from build123d import *

# Parameters (mm, degrees)
SKIZZE1_R                            = 33.5
AUFSATZ_LINEAR_AUSTRAGEN1_DEPTH      = 36
SKIZZE2_R                            = 19
AUFSATZ_LINEAR_AUSTRAGEN2_DEPTH      = 4.5
SKIZZE3_R                            = 13.25
AUFSATZ_LINEAR_AUSTRAGEN3_DEPTH      = 6
SKIZZE4_R                            = 13
AUFSATZ_LINEAR_AUSTRAGEN4_DEPTH      = 26
AUFSATZ_LINEAR_AUSTRAGEN4_DEPTH_BACK = 29
SKIZZE5_R                            = 20
AUFSATZ_LINEAR_AUSTRAGEN5_DEPTH      = 9
SKIZZE6_R                            = 31.75
AUFSATZ_LINEAR_AUSTRAGEN6_DEPTH      = 7
SKIZZE7_W                            = 58.3
SKIZZE7_H                            = 58.3
AUFSATZ_LINEAR_AUSTRAGEN7_DEPTH      = 7
F_10_0_10_DURCHMESSER_BOHRUNG1_D     = 10
F_10_0_10_DURCHMESSER_BOHRUNG1_DEPTH = 7
SKIZZE13_R                           = 19
AUFSATZ_LINEAR_AUSTRAGEN8_DEPTH      = 4.5
SKIZZE14_R                           = 13.25
AUFSATZ_LINEAR_AUSTRAGEN9_DEPTH      = 6
SKIZZE15_R                           = 6
AUFSATZ_LINEAR_AUSTRAGEN10_DEPTH     = 55
SKIZZE16_R                           = 6
AUFSATZ_LINEAR_AUSTRAGEN11_DEPTH     = 55


with BuildPart() as part:
    # Skizze1 → Aufsatz-Linear austragen1 (new body)
    with BuildSketch(Plane.XY):
        Circle(SKIZZE1_R)
    extrude(amount=AUFSATZ_LINEAR_AUSTRAGEN1_DEPTH)

    # Skizze2 → Aufsatz-Linear austragen2 (add)
    with BuildSketch(Plane.XY.offset(36)):
        Circle(SKIZZE2_R)
    extrude(amount=AUFSATZ_LINEAR_AUSTRAGEN2_DEPTH)

    # Skizze3 → Aufsatz-Linear austragen3 (add)
    with BuildSketch(Plane.XY.offset(40.5)):
        Circle(SKIZZE3_R)
    extrude(amount=AUFSATZ_LINEAR_AUSTRAGEN3_DEPTH)

    # Skizze4 → Aufsatz-Linear austragen4 (add, two sides)
    with BuildSketch(Plane(origin=(0, 0, 0), x_dir=(1, 0, 0), z_dir=(0, 1, 0))) as aufsatz_linear_austragen4_sk:
        with Locations((-33.5, -18)):
            Circle(SKIZZE4_R)
    extrude(amount=AUFSATZ_LINEAR_AUSTRAGEN4_DEPTH)
    extrude(aufsatz_linear_austragen4_sk.sketch, amount=-AUFSATZ_LINEAR_AUSTRAGEN4_DEPTH_BACK)

    # Skizze5 → Aufsatz-Linear austragen5 (add)
    with BuildSketch(Plane(origin=(0, 26, 0), x_dir=(1, 0, 0), z_dir=(0, 1, 0))):
        with Locations((-33.5, -18)):
            Circle(SKIZZE5_R)
    extrude(amount=AUFSATZ_LINEAR_AUSTRAGEN5_DEPTH)

    # Skizze6 → Aufsatz-Linear austragen6 (add)
    with BuildSketch(Plane(origin=(0, 35, 0), x_dir=(1, 0, 0), z_dir=(0, 1, 0))):
        with Locations((-33.5, -18)):
            Circle(SKIZZE6_R)
    extrude(amount=AUFSATZ_LINEAR_AUSTRAGEN6_DEPTH)

    # Skizze7 → Aufsatz-Linear austragen7 (add)
    with BuildSketch(Plane(origin=(0, 42, 0), x_dir=(1, 0, 0), z_dir=(0, 1, 0))):
        with Locations((-33.5, -18)):
            Rectangle(SKIZZE7_W, SKIZZE7_H)
    extrude(amount=-AUFSATZ_LINEAR_AUSTRAGEN7_DEPTH)

    # Ø10.0 (10) Durchmesser Bohrung1
    with Locations(Plane(origin=(0, 42, 0), x_dir=(1, 0, 0), z_dir=(0, 1, 0))):
        with Locations((-57.5, -42), (-57.5, 6), (-9.5, 6), (-9.5, -42)):
            Hole(F_10_0_10_DURCHMESSER_BOHRUNG1_D / 2, depth=F_10_0_10_DURCHMESSER_BOHRUNG1_DEPTH)

    # Skizze13 → Aufsatz-Linear austragen8 (add)
    with BuildSketch(Plane(origin=(0, 0, 0), x_dir=(-1, 0, 0), z_dir=(0, 0, -1))):
        Circle(SKIZZE13_R)
    extrude(amount=AUFSATZ_LINEAR_AUSTRAGEN8_DEPTH)

    # Skizze14 → Aufsatz-Linear austragen9 (add)
    with BuildSketch(Plane(origin=(0, 0, -4.5), x_dir=(-1, 0, 0), z_dir=(0, 0, -1))):
        Circle(SKIZZE14_R)
    extrude(amount=AUFSATZ_LINEAR_AUSTRAGEN9_DEPTH)

    # Skizze15 → Aufsatz-Linear austragen10 (add)
    with BuildSketch(Plane(origin=(0, 0, -10.5), x_dir=(-1, 0, 0), z_dir=(0, 0, -1))):
        Circle(SKIZZE15_R)
    extrude(amount=AUFSATZ_LINEAR_AUSTRAGEN10_DEPTH)

    # Skizze16 → Aufsatz-Linear austragen11 (add)
    with BuildSketch(Plane.XY.offset(46.5)):
        Circle(SKIZZE16_R)
    extrude(amount=AUFSATZ_LINEAR_AUSTRAGEN11_DEPTH)


solid = part.part
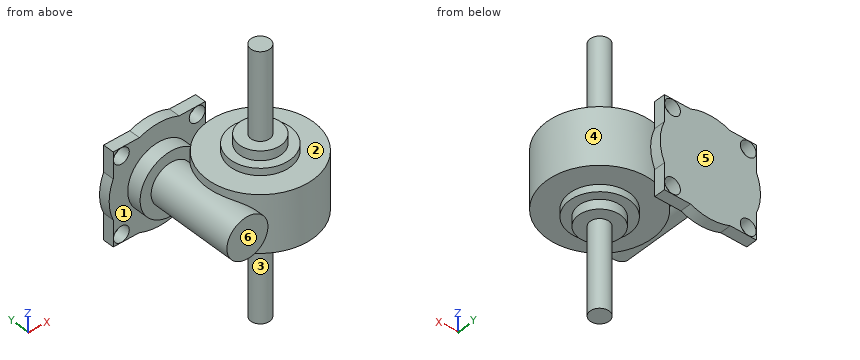
Design review of the part built by this model. Coordinates are the model's own, in mm. Face numbers are marked on the shaded views. A direction names the side the tool comes from. Round coordinates to 2 decimals unless told otherwise and drop trailing zeros. Write each loop counter-clockwise with the first axis right and the second up, starting at its lowest first coordinate (ties: lowest second). Pieces come first, ordered by that corner, then holes. Notation, with made-up numbers: (-14.75, 61) -> (23.25, 61) arc R16 cw to (23.25, 79) -> close; hole circle Ø8 at (12, -18). An arc over 180 degrees is marked (long way). One line per item, written item: value. Start each with the question number.
Q1. To check wall thickness, follow probe 1 along Z at (x, y) = (-57.5, 38.5); probe 2 along Z at (x, y) = (-10, 2); probe 3 along Z at (x, y) = (1, -17.5). State the ranges of each line that lie inside material, in increasing order.
Q2. Add section B-B (x = 0.5). Give the boundary of the cut face in (y, z), then the cut area to 3 significant figures.
Q3. Add section D-D (z = -22). Give the boundary of the cut face in (x, y).
Q4. Tool access review of the marked faces 1, 2 and 3: name each direction out of +Z, -Z, +X, -X, +Y, -Y from which nothing blocks a thin tool from reaching the whole face with its end or side.
Q5. Add section C-C (y = 21.5). Give the boundary of the cut face in (x, z), then the cut area to 3 significant figures.
Q6. Insertion check: P1, Ø6, axis at x = -9.5, z = -6, coming from the +Y side; P2, Ø3.5, axis at x = -14.5, y = 40, coming from the +Z side; P3, Ø5.5, axis at y = 37.5, z = 41, coming from the -X side. Each pin has a flat end and moves straight along its axis. Give the tip position at first contact, or say it passes through.
Q7. The part is to be moulded in two halves that separate along Y. For the marked faces 4, 5 and 6, say which applies: pulls with the +Y half, pulls with the -Y half, needs draft (parallel to the pull), parting line crosses it, or undercut.
Q8. Add section A-A (x = -9.5). State how many separate pieces and enclosed holes the cut face has, then the cut area to 3 significant figures.
Response:
1. probe 1: z = -11.15 to -11, -1 to 37, 47 to 47.15
1. probe 2: z = -10.5 to 46.5
1. probe 3: z = -4.5 to 40.5
2. outline: (-33.5, 0) -> (-18.99, 0) -> (-18.99, -4.5) -> (-13.24, -4.5) -> (-13.24, -10.5) -> (-5.98, -10.5) -> (-5.98, -65.5) -> (5.98, -65.5) -> (5.98, -10.5) -> (13.24, -10.5) -> (13.24, -4.5) -> (18.99, -4.5) -> (18.99, 0) -> (33.5, 0) -> (33.5, 36) -> (18.99, 36) -> (18.99, 40.5) -> (13.24, 40.5) -> (13.24, 46.5) -> (5.98, 46.5) -> (5.98, 101.5) -> (-5.98, 101.5) -> (-5.98, 46.5) -> (-13.24, 46.5) -> (-13.24, 40.5) -> (-18.99, 40.5) -> (-18.99, 36) -> (-33.5, 36) -> close
2. area: 4,390 mm^2
3. outline: circle Ø12 at (0, 0)
4. face 1: none
4. face 2: +Z
4. face 3: -Z
5. outline: (-25.69, 0) -> (25.69, 0) -> (25.69, 36) -> (-25.69, 36) -> (-25.69, 28.39) arc R13 ccw (long way) to (-25.69, 7.61) -> close
5. area: 2,310 mm^2
6. P1: stops at y = 17.7
6. P2: stops at z = 47.15
6. P3: stops at x = -62.65
7. face 4: undercut
7. face 5: pulls with the +Y half
7. face 6: pulls with the -Y half
8. separate pieces: 4
8. enclosed holes: 0
8. area: 3,100 mm^2
